The drawing under review shows one solid part. Ordinate dimensions are in mm from its lowest x, y, z. A direction names the side the tool comes from. Coordinates: 2 decimals unless noted, no trailing zeros. Loops run counter-clockwise (first coordinate to the right, second up) from the corner with the lowest first, then second, coordinate; pieces in that order, holes last. Notation, with made-up numbers: (57.25, -37.5) - (83.25, -37.5) arc R26 cw to (83.25, -3.5) - close; hole circle Ø8 at (74, 34). An arc over 180 degrees is marked (long way). Use one line per item in the form item = value. Start each with the question number.
1. Add section C-C on z = 49. Give the boundary of the cut face in (x, y) (3 decimals).
2. Machinability: for the marked faces 1 and 2, which of the approach directions +Z, -Z, +X, -X, +Y, -Y give a long, thin tool a straight path to every point of the face, cutting with its end or side? Answer none if there is none.
3. For pin 1 Ø4 at (x, z) = (42.5, 14) entering from +Y; pin 2 Ø1 at (x, z) = (9, 61) entering from -Y, all flat-tipped, find the tip position at first contact; note any pin that passes through.
4. Add section A-A on z = 5.5. Give the boundary of the cut face in (x, y), and give its area (3 significant figures).
5. Add section B-B on x = 25. Give the boundary of the cut face in (y, z) (1 decimal), and give its area (3 significant figures).
6. To check wall thickness, follow probe 1 along Z at (x, y) = (33, 46); probe 2 along X at (y, z) = (12, 4.5). State the ranges of each line that lie inside material, in increasing order.
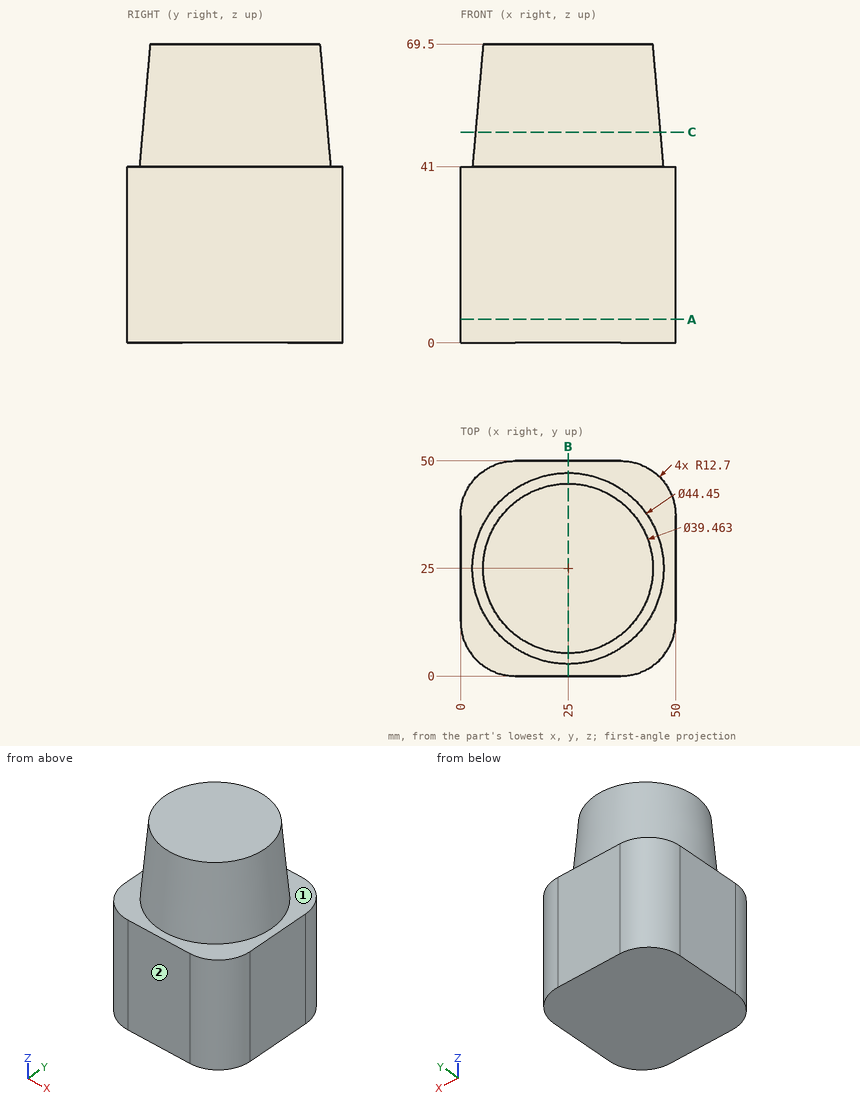
Conclusion:
q1.outline = circle Ø43.05 at (25, 25)
q2.face_1 = +Z
q2.face_2 = +Z, -Z, +X, -X, -Y
q3.pin_1 = 49.59
q3.pin_2 = 11.62
q4.outline = (0, 12.7) arc R12.7 ccw to (12.7, 0) - (37.3, 0) arc R12.7 ccw to (50, 12.7) - (50, 37.3) arc R12.7 ccw to (37.3, 50) - (12.7, 50) arc R12.7 ccw to (0, 37.3) - close
q4.area = 2,360 mm^2
q5.outline = (0, 0) - (50, 0) - (50, 41) - (47.2, 41) - (44.7, 69.5) - (5.3, 69.5) - (2.8, 41) - (0, 41) - close
q5.area = 3,250 mm^2
q6.probe_1 = 0 to 41
q6.probe_2 = 0.02 to 49.98
